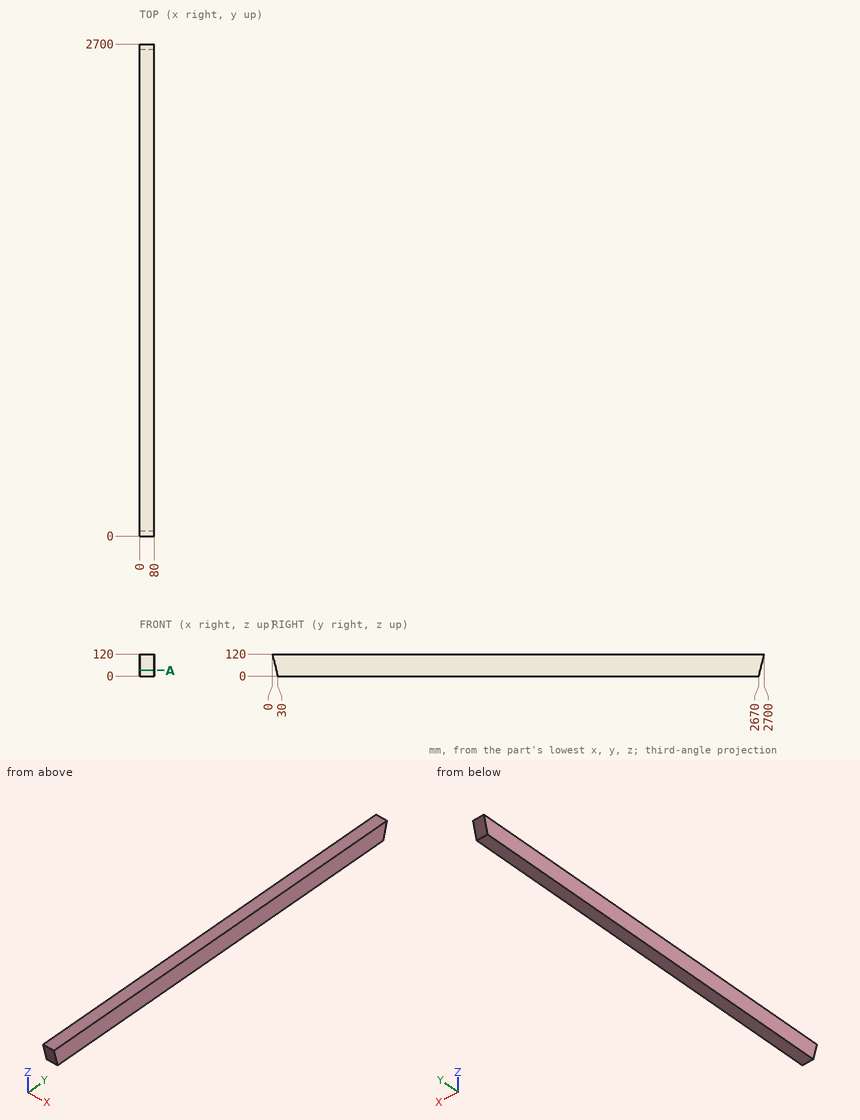
Verification items for this drawing (mm, ordinates from the low corner). Coordinates: 2 decimals unless noted, no trailing zeros. Order: outer loops, then holes, each group sorted by start corner. A loop starts at its lowest first (then second) coordinate and runs counter-clockwise, first axis right, second up.
Q1. Depth check by flat-ended pin: pin 1 Ø5 at (x, z) = (27, 23.5) entering from -Y; pin 2 Ø1 at (x, z) = (22, 35.5) entering from -Y; pin 3 Ø12 at (x, z) = (37.5, 55.5) entering from -Y (3 decimals); pin 4 Ø5 at (y, z) = (2374.5, 65.5) entering from -X. Enter the tip coordinate at first touch or a pass-through.
Reply:
pin 1: stops at y = 23.5
pin 2: stops at y = 21
pin 3: stops at y = 14.625
pin 4: stops at x = 0
Q2. Thickness scan on probe 1 along Y at (x, z) = (22.5, 36); probe 2 along Y at (x, z) = (77, 77.5) (3 decimals). Record the ranges inside material, lowest first.
Reply:
probe 1: y = 21 to 2679
probe 2: y = 10.625 to 2689.375
Q3. Sectioned sample at A-A on z = 31. Record the cut outline in (x, y).
Reply:
outline: (0, 22.25) - (80, 22.25) - (80, 2677.75) - (0, 2677.75) - close
